Job drawing, mm, ordinate dimensions from the low corner. One solid piece. Round coordinates to 2 decimals unless told otherwise and drop trailing zeros. Loops run counter-clockwise (first coordinate to the right, second up) from the corner with the lowest first, then second, coordinate; pieces in that order, holes last.
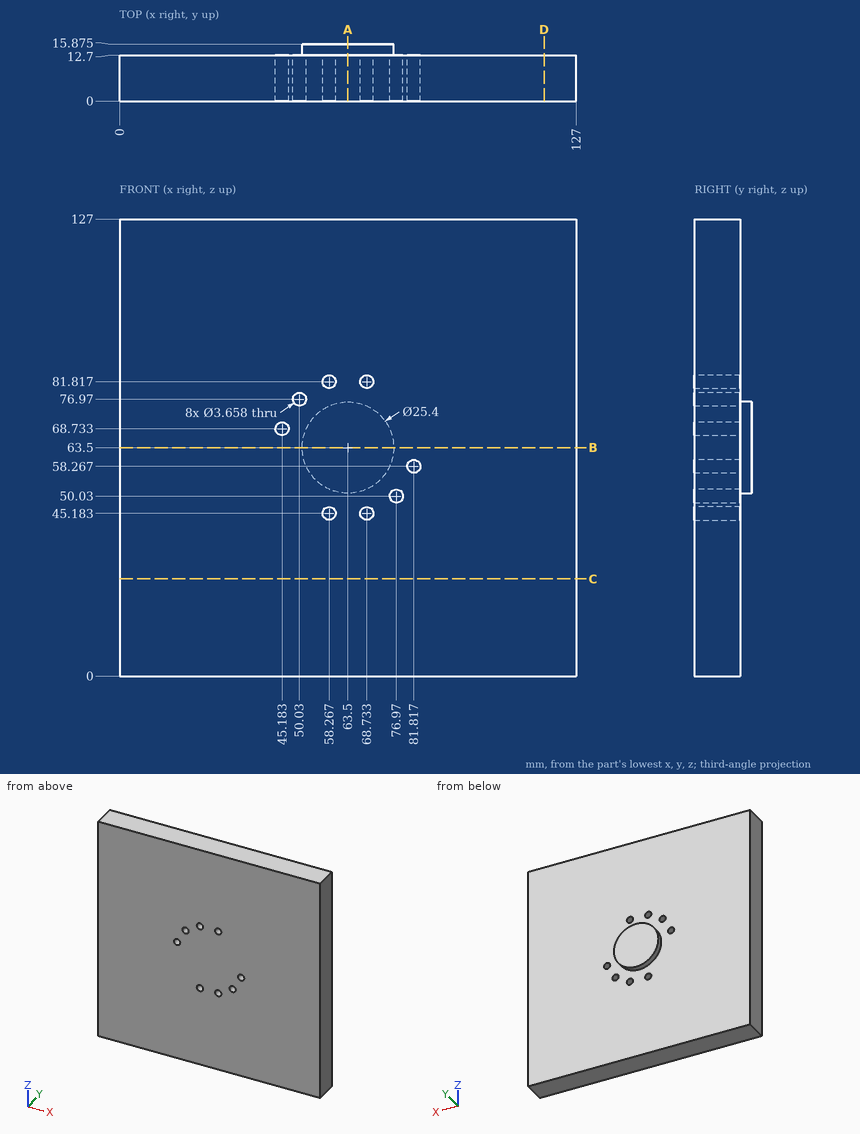
Item 1: Cut at A-A, the plane x = 63.5. Give the cut face in (y, z) (1 decimal).
Answers follow:
outline: (0, 0) - (12.7, 0) - (12.7, 50.8) - (15.9, 50.8) - (15.9, 76.2) - (12.7, 76.2) - (12.7, 127) - (0, 127) - close
Item 2: Flat gauge pins, fed straight in: P1, Ø4, axis at x = 58.27, z = 81.82, coming from the +Y side; P2, Ø3, axis at x = 58.27, z = 45.18, coming from the +Y side. Where does each tip first touch, or does it go through?
Answers follow:
P1: stops at y = 12.7
P2: passes through
Item 3: Cut at C-C, the plane z = 27. Give the cut face in (x, y), plus the area to 3 significant figures.
Answers follow:
outline: (0, 0) - (127, 0) - (127, 12.7) - (0, 12.7) - close
area: 1,610 mm2
Item 4: Cut at B-B, the plane z = 63.5. Give the cut face in (x, y) (1 decimal).
Answers follow:
outline: (0, 0) - (127, 0) - (127, 12.7) - (76.2, 12.7) - (76.2, 15.9) - (50.8, 15.9) - (50.8, 12.7) - (0, 12.7) - close
Item 5: Probe line 1 (Z direction, x = 69, y = 12); line 2 (Z direction, x = 50, y = 3.25); line 3 (Y direction, x = 70, z = 28). List the from-to ranges inside material, lowest first.
Answers follow:
line 1: z = 0 to 43.37, 46.99 to 80.01, 83.63 to 127
line 2: z = 0 to 75.14, 78.8 to 127
line 3: y = 0 to 12.7
Item 6: Cut at D-D, the plane x = 118. Give the cut face in (y, z).
Answers follow:
outline: (0, 0) - (12.7, 0) - (12.7, 127) - (0, 127) - close
